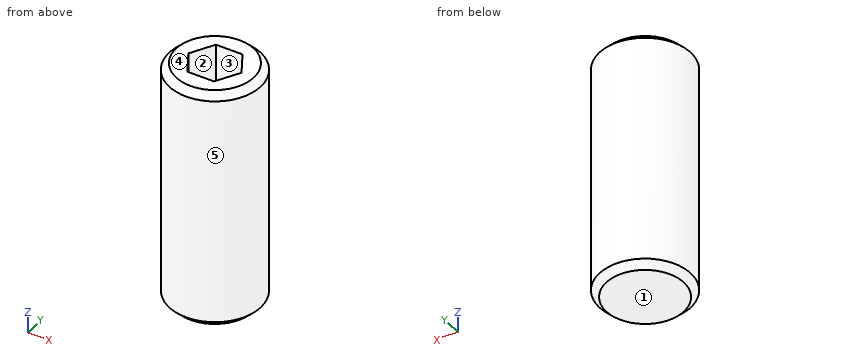
Solid Edge part; units mm, degrees
sketch "Sketch1" plane through (0, 0, 0) normal (0, 0, 1) x (1, 0, 0)
  circle A0 centre (0, 0) radius 3
extrude "Protrusion1" add sketch "Sketch1" along normal mid plane 16
chamfer "Chamfer1" distance 0.45 angle 45 2 edges at (-3, 0, -8) (-3, 0, 8)
sketch "Sketch2" plane through (0, 0, 8) normal (0, 0, 1) x (1, 0, 0)
  line L0 (-0.866, 1.5) -> (0.866, 1.5)
  line L1 (1.7321, 0) -> (0.866, 1.5)
  line L2 (0.866, -1.5) -> (1.7321, 0)
  line L3 (-0.866, -1.5) -> (0.866, -1.5)
  line L4 (-1.7321, 0) -> (-0.866, -1.5)
  line L5 (-0.866, 1.5) -> (-1.7321, 0)
extrude "Cutout1" cut sketch "Sketch2" against normal blind 8
properties part number "24104725"
Part model, mm, in its own coordinate system. Face numbers are marked on the shaded views. A direction names the side the tool comes from. Coordinates: 2 decimals unless noted, no trailing zeros. Order: outer loops, then holes, each group sorted by start corner. A loop starts at its lowest first (then second) coordinate and runs counter-clockwise, first axis right, second up. Notation, with made-up numbers: (-36.5, 80) -> (-0.5, 80) arc R25 cw to (-0.5, 97) -> close; hole circle Ø11 at (-4.75, 70). An arc over 180 degrees is marked (long way). Put each result on its own line as item: value. Start each with the question number.
(1) Which spindle directions (+Z, -Z, +X, -X, +Y, -Y) get a long thin tool onto all of the face, cutting with end or side? Do the marked faces 1 and 2. Say none if no direction does.
(2) Band-saw the part on C-C (z = -6.25). Give the cut face in (x, y), then the cut area to 3 significant figures.
(3) Pin check, flat tips, straight feed: pin 1 Ø2 at (x, z) = (-2.5, 0) entering from +Y; pin 2 Ø2 at (x, z) = (1.5, 3.5) entering from +Y; pin 3 Ø1 at (y, z) = (1, 1.5) entering from -X. Stop position of each tip, or through.
(4) Band-saw the part on B-B (x = 0). Give the cut face in (y, z), then the cut area to 3 significant figures.
(5) Probe line 1 along Z through (x, y) = (-1.05, -0.8); line 2 along Y through (x, z) = (2.6, 6.75); line 3 along X through (y, z) = (2.45, 3.25). List the from-to ranges inside material, lowest first. Write a range as [from, to].
(6) Mould opens along Y. For the marked faces 3, 4 and 5 say: pulls with the +Y half, pulls with the -Y half, needs draft (parallel to the pull), parting line crosses it, or undercut.
(7) Band-saw the part on A-A (z = 7). Give the cut face in (x, y).
Determined:
1. face 1: -Z, +X, -X, +Y, -Y
1. face 2: +Z
2. outline: circle Ø6 at (0, 0)
2. area: 28.3 mm²
3. pin 1: stops at y = 2.6
3. pin 2: stops at y = 2.96
3. pin 3: stops at x = -2.96
4. outline: (-3, -7.55) -> (-2.55, -8) -> (2.55, -8) -> (3, -7.55) -> (3, 7.55) -> (2.55, 8) -> (1.5, 8) -> (1.5, 0) -> (-1.5, 0) -> (-1.5, 8) -> (-2.55, 8) -> (-3, 7.55) -> close
4. area: 71.6 mm²
5. line 1: z = [-8, 0]
5. line 2: y = [-1.5, 1.5]
5. line 3: x = [-1.73, 1.73]
6. face 3: undercut
6. face 4: needs draft
6. face 5: parting line crosses it
7. outline: circle Ø6 at (0, 0); hole (-1.73, 0) -> (-0.87, -1.5) -> (0.87, -1.5) -> (1.73, 0) -> (0.87, 1.5) -> (-0.87, 1.5) -> close
